```python
from build123d import *

# Parameters (mm, degrees)
BOSS_EXTRUDE1_DEPTH            = 32
CBORE_FOR_M3_SHCS1_D           = 4.9
CBORE_FOR_M3_SHCS1_CBORE_D     = 5.5
CBORE_FOR_M3_SHCS1_CBORE_DEPTH = 0.5


with BuildPart() as part:
    # Sketch1 → Boss-Extrude1 (new, symmetric)
    with BuildSketch(Plane.XY):
        with BuildLine():
            Line((-20.6, 0), (-12.6, 0))
            ThreePointArc((-12.6, 0), (0, 12.6), (12.6, 0))
            Line((12.6, 0), (20.6, 0))
            ThreePointArc((20.6, 0), (0, 20.6), (-20.6, 0))
        make_face()
    extrude(amount=BOSS_EXTRUDE1_DEPTH, both=True)

    # CBORE for M3 SHCS1 (through all)
    with Locations(Plane.XZ):
        with Locations((-16.6, -25), (16.6, 25), (-16.6, 25), (16.6, -25)):
            CounterBoreHole(CBORE_FOR_M3_SHCS1_D / 2, CBORE_FOR_M3_SHCS1_CBORE_D / 2, CBORE_FOR_M3_SHCS1_CBORE_DEPTH)


solid = part.part
```
The listing builds one solid part. Answer for the finished solid, in the listing's coordinates (mm). A direction names the side the tool comes from. Coordinates: 2 decimals unless noted, no trailing zeros. Loops run counter-clockwise (first coordinate to the right, second up) from the corner with the lowest first, then second, coordinate; pieces in that order, holes last. Notation, with made-up numbers: (50.25, -22.75) -> (90.25, -22.75) arc R35 ccw to (90.25, 13.25) -> close; hole circle Ø10 at (-13, -9.75). An arc over 180 degrees is marked (long way). Use one line per item in the form item = value. Start each with the question number.
Item 1: The part is cut by section D-D on y = 1.5. Determine the outline of the cut face in (x, z), then the cut area to 3 significant figures.
Item 2: The part is cut by section A-A on y = 6.75. Determine the outline of the cut face in (x, z), then the cut area to 3 significant figures.
Item 3: A tool of negligible diameter and unlimited length cuts with its end or side. For faces 4 (the face through (-16.958, 0.246, -22.273)), 5 (the face through (-17, 0, 0)), from which of +Z, -Z, +X, -X, +Y, -Y can it reach the whole face along a straight path? Write none if from no direction.
Item 4: Consider L1, parallel to Z at x = 16.6, y = 0.2; L2, parallel to Z at x = -16.6, y = 9.25; L3, parallel to X at y = 7.5, z = 7. Determine where each line is inside the solid, lowest interval first. Write a range as [from, to].
Item 5: The part is cut by section B-B on z = 26.5. Determine the outline of the cut face in (x, y), then the cut area to 3 significant figures.
Item 6: The part is cut by section C-C on x = 16.6. Determine the outline of the cut face in (y, z), then the cut area to 3 significant figures.
Item 7: Flat-ended cylindrical pins translate along their axes: pin 1 Ø9 at (x, z) = (-16.6, -25) entering from +Y; pin 2 Ø10 at (y, z) = (3.5, -4) entering from +X; pin 3 Ø5.5 at (x, z) = (-16.6, -25) entering from +Y; pin 4 Ø4.5 at (x, z) = (-16.6, 25) entering from -Y. Find the tip coordinate at first contact, or state that the pin passes through.
Item 8: The mould has two halves that part along X. Classify faces 1 (the face through (0.453, 20.595, 0.448)), 2 (the face through (17, 0, 0)), 3 (the face through (-14.152, 6.229, 25.108)): released by +X, released by -X, zero draft, split by the parting line, or undercut.
Answer key:
q1.outline = (-20.55, -32) -> (-12.51, -32) -> (-12.51, 32) -> (-20.55, 32) -> close; (12.51, -32) -> (20.55, -32) -> (20.55, 32) -> (12.51, 32) -> close; hole circle Ø4.9 at (-16.6, -25); hole circle Ø4.9 at (-16.6, 25); hole circle Ø4.9 at (16.6, -25); hole circle Ø4.9 at (16.6, 25)
q1.area = 953 mm2
q2.outline = (-19.46, -32) -> (-10.64, -32) -> (-10.64, 32) -> (-19.46, 32) -> close; (10.64, -32) -> (19.46, -32) -> (19.46, 32) -> (10.64, 32) -> close; hole circle Ø4.9 at (-16.6, -25); hole circle Ø4.9 at (-16.6, 25); hole circle Ø4.9 at (16.6, -25); hole circle Ø4.9 at (16.6, 25)
q2.area = 1,050 mm2
q3.face_4 = -Y
q3.face_5 = +Z, -Z, +X, -X, -Y
q4.L1 = [-32, -27.75], [-22.25, 22.25], [27.75, 32]
q4.L2 = [-32, -27.45], [-22.55, 22.55], [27.45, 32]
q4.L3 = [-19.19, -10.12], [10.12, 19.19]
q5.outline = (-20.6, 0) -> (-18.9, 0) -> (-18.9, 0.5) -> (-18.54, 0.5) -> (-18.54, 8.99) arc R20.6 ccw to start; (-14.66, 0.5) -> (-14.3, 0.5) -> (-14.3, 0) -> (-12.6, 0) arc R12.6 cw to (12.6, 0) -> (14.3, 0) -> (14.3, 0.5) -> (14.66, 0.5) -> (14.66, 14.47) arc R20.6 ccw to (-14.66, 14.47) -> close; (18.54, 0.5) -> (18.9, 0.5) -> (18.9, 0) -> (20.6, 0) arc R20.6 ccw to (18.54, 8.99) -> close
q5.area = 323 mm2
q6.outline = (0, -32) -> (12.2, -32) -> (12.2, -27.45) -> (0.5, -27.45) -> (0.5, -27.75) -> (0, -27.75) -> close; (0, -22.25) -> (0.5, -22.25) -> (0.5, -22.55) -> (12.2, -22.55) -> (12.2, 22.55) -> (0.5, 22.55) -> (0.5, 22.25) -> (0, 22.25) -> close; (0, 27.75) -> (0.5, 27.75) -> (0.5, 27.45) -> (12.2, 27.45) -> (12.2, 32) -> (0, 32) -> close
q6.area = 661 mm2
q7.pin_1 = 16.67
q7.pin_2 = 20.6
q7.pin_3 = 15.25
q7.pin_4 = through
q8.face_1 = split by the parting line
q8.face_2 = zero draft
q8.face_3 = undercut
